Can you work these out from the model? Positions are in its coordinate system, mm. A direction names the side the tool comes from. Coordinates: 2 decimals unless noted, no trailing zeros. Order: outer loops, then holes, each group sorted by start corner. A loop starts at its lowest first (then second) coordinate and runs counter-clockwise, first axis right, second up. Notation, with made-up numbers: (19.5, 39) - (67.5, 39) arc R33 ccw to (67.5, 75) - close; hole circle Ø11 at (68, 20.5). An arc over 180 degrees is marked (long way). Use a Markdown table: item, result. Add a question column.
(1) For pin 1 Ø1.2 at (x, z) = (44, 1.5) entering from -Y; pin 2 Ø1.2 at (x, z) = (45.5, 2) entering from +Y; pin 3 Ø3 at (x, y) = (-30.5, 0) entering from +Z, each with a flat end and sliding along its axis, tell me the tip position at first contact or that it passes through.
(2) I want a section at C-C (y = -30). List the corners of the cut face in (x, z) for me.
(3) We'd pull the mould along Y, two halves only. Please class faces 1 (the flat face through (42, 20, 2)), 2 (the flat face through (42.5, 0, 2)), 3 (the flat face through (-42, -20, 2)): pulls with the +Y half, pulls with the -Y half, needs draft (parallel to the pull), parting line crosses it, or undercut.
(4) I want a section at B-B (x = 0). List the corners of the cut face in (y, z) for me.
(5) If I drill on L1, parallel to Y at x = 0, z = 2.05; L2, parallel to X at y = -7, z = 3.35; L3, parallel to Y at x = -43, z = 1.2, over which ranges is the centre line in solid material (lowest first)? Write a range as [from, to].
(6) I want a section at A-A (y = 7.5). List the corners of the cut face in (x, z) for me, and give its area (3 significant figures).
(7) On a 3-axis mill with a long thin cutter (end or side, diameter ignored), from which of +Z, -Z, +X, -X, +Y, -Y can I reach the whole of each face in a straight line? I mean faces 4 (the cylindrical face through (34.87, 20.38, 2.03)), 5 (the flat face through (30, 0, 1.3)), 6 (the flat face through (42, -20, 2)). Say none if no direction works.
```python
from build123d import *

# Parameters (mm, degrees)
BOSS_EXTRU_1_DEPTH           = 4
ESQUISSE2_R                  = 3.1
ENL_V_MAT_EXTRU_1_DEPTH      = 1
ENL_V_MAT_EXTRU_1_DEPTH_BACK = 2.7
ESQUISSE3_W                  = 5
ESQUISSE3_H                  = 30
ENL_V_MAT_EXTRU_2_DEPTH      = 12.7
CONG_1_R                     = 1.5
CONG_2_R                     = 3
CONG_3_R                     = 3


with BuildPart() as part:
    # Esquisse1 → Boss.-Extru.1 (new body)
    with BuildSketch(Plane.XY):
        with BuildLine():
            Line((-34.641016151, -20), (-50, -20))
            Line((-50, -20), (-50, 20))
            Line((-50, 20), (-34.641016151, 20))
            ThreePointArc((-34.641016151, 20), (0, 40), (34.641016151, 20))
            Line((34.641016151, 20), (50, 20))
            Line((50, 20), (50, -20))
            Line((50, -20), (34.641016151, -20))
            ThreePointArc((34.641016151, -20), (0, -40), (-34.641016151, -20))
        make_face()
    extrude(amount=BOSS_EXTRU_1_DEPTH)

    # Esquisse2 → Enlèv. mat.-Extru.1 (cut, two sides)
    with BuildSketch(Plane.XY.offset(4)) as enl_v_mat_extru_1_sk:
        with Locations((0, 30)):
            Circle(ESQUISSE2_R)
        with Locations((30, 0)):
            Circle(ESQUISSE2_R)
        with Locations((0, -30)):
            Circle(ESQUISSE2_R)
        with Locations((-30, 0)):
            Circle(ESQUISSE2_R)
    extrude(amount=ENL_V_MAT_EXTRU_1_DEPTH, mode=Mode.SUBTRACT)
    extrude(enl_v_mat_extru_1_sk.sketch, amount=-ENL_V_MAT_EXTRU_1_DEPTH_BACK, mode=Mode.SUBTRACT)

    # Esquisse3 → Enlèv. mat.-Extru.2 (cut)
    with BuildSketch(Plane.XY.offset(4)):
        with Locations((-45, 0)):
            Rectangle(ESQUISSE3_W, ESQUISSE3_H)
        with Locations((45, 0)):
            Rectangle(ESQUISSE3_W, ESQUISSE3_H)
    extrude(amount=-ENL_V_MAT_EXTRU_2_DEPTH, mode=Mode.SUBTRACT)

    # Congé1
    cong_1_edges = [part.edges().sort_by_distance(p)[0] for p in [
        (47.5, 0, 0),
        (-47.5, 0, 0),
        (-47.5, 0, 4),
        (47.5, 0, 4),
    ]]
    fillet(cong_1_edges, radius=CONG_1_R)

    # Congé2
    cong_2_edges = [part.edges().sort_by_distance(p)[0] for p in [
        (50, 20, 2),
        (50, -20, 2),
        (-50, -20, 2),
        (-50, 20, 2),
    ]]
    fillet(cong_2_edges, radius=CONG_2_R)

    # Congé3
    cong_3_edges = [part.edges().sort_by_distance(p)[0] for p in [
        (34.641016151, 20, 2),
        (34.641016151, -20, 2),
        (-34.641016151, -20, 2),
        (-34.641016151, 20, 2),
    ]]
    fillet(cong_3_edges, radius=CONG_3_R)


solid = part.part
```
Answers follow:
| question | item | result |
|---|---|---|
| 1 | pin 1 | stops at y = -20 |
| 1 | pin 2 | stops at y = 20 |
| 1 | pin 3 | stops at z = 1.3 |
| 2 | outline | (-26.46, 0) - (26.46, 0) - (26.46, 4) - (3.1, 4) - (3.1, 1.3) - (-3.1, 1.3) - (-3.1, 4) - (-26.46, 4) - close |
| 3 | face 1 | pulls with the +Y half |
| 3 | face 2 | undercut |
| 3 | face 3 | pulls with the -Y half |
| 4 | outline | (-40, 0) - (40, 0) - (40, 4) - (33.1, 4) - (33.1, 1.3) - (26.9, 1.3) - (26.9, 4) - (-26.9, 4) - (-26.9, 1.3) - (-33.1, 1.3) - (-33.1, 4) - (-40, 4) - close |
| 5 | L1 | y = [-40, -33.1], [-26.9, 26.9], [33.1, 40] |
| 5 | L2 | x = [-50, -47.76], [-42.5, 42.5], [47.76, 50] |
| 5 | L3 | y = [-20, -15], [15, 20] |
| 6 | outline | (-50, 0) - (-49, 0) arc R1.5 ccw to (-47.5, 1.5) - (-47.5, 2.5) arc R1.5 ccw to (-49, 4) - (-50, 4) - close; (-42.5, 0) - (42.5, 0) - (42.5, 4) - (-42.5, 4) - close; (47.5, 1.5) arc R1.5 ccw to (49, 0) - (50, 0) - (50, 4) - (49, 4) arc R1.5 ccw to (47.5, 2.5) - close |
| 6 | area | 358 mm² |
| 7 | face 4 | +Z, -Z, +X, +Y |
| 7 | face 5 | +Z |
| 7 | face 6 | +Z, -Z, +X, -Y |
